Geometry: final body of the model. Coordinates: model frame, mm. Coordinates: 2 decimals unless noted, no trailing zeros. Write each loop counter-clockwise with the first axis right and the second up, starting at its lowest first coordinate (ties: lowest second). Pieces come first, ordered by that corner, then holes. Notation, with made-up numbers: (-9, 52.5) -> (34, 52.5) arc R17 ccw to (34, 83.5) -> close; hole circle Ø6 at (66, 74). An arc over 180 degrees is marked (long way). Answer as a JSON object with one key per item and string values. Group by question number.
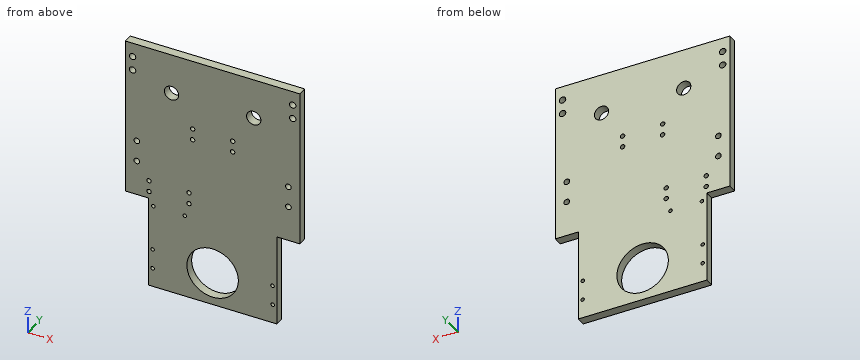
```python
from build123d import *

# Parameters (mm, degrees)
SKETCH1_W           = 122
SKETCH1_H           = 112
BOSS_EXTRUDE1_DEPTH = 6.2
SKETCH2_W           = 90
SKETCH2_H           = 65
BOSS_EXTRUDE2_DEPTH = 6.2
SKETCH3_R           = 1.25
SKETCH3_R_2         = 18
CUT_EXTRUDE1_DEPTH  = 136.648221514
SKETCH4_R           = 1.55
CUT_EXTRUDE2_DEPTH  = 136.648221514
SKETCH5_R           = 2
CUT_EXTRUDE3_DEPTH  = 10
SKETCH6_R           = 5
CUT_EXTRUDE4_DEPTH  = 10
SKETCH7_R           = 2.25
CUT_EXTRUDE5_DEPTH  = 136.648221514


with BuildPart() as part:
    # Sketch1 → Boss-Extrude1 (new body)
    with BuildSketch(Plane(origin=(0, 0, 0), x_dir=(1, 0, 0), z_dir=(0, 1, 0))):
        Rectangle(SKETCH1_W, SKETCH1_H)
    extrude(amount=BOSS_EXTRUDE1_DEPTH)

    # Sketch2 → Boss-Extrude2 (add)
    with BuildSketch(Plane(origin=(0, 0, 0), x_dir=(1, 0, 0), z_dir=(0, 1, 0))):
        with Locations((0, 88.5)):
            Rectangle(SKETCH2_W, SKETCH2_H)
    extrude(amount=BOSS_EXTRUDE2_DEPTH)

    # Sketch3 → Cut-Extrude1 (cut, through all)
    with BuildSketch(Plane(origin=(0, 6.2, 0), x_dir=(1, 0, 0), z_dir=(0, 1, 0))):
        with Locations(Location((-41.5, 61, 0), (0, 0, 270))):
            Circle(SKETCH3_R)
        with Locations(Location((-19.5, 61, 0), (0, 0, 270))):
            Circle(SKETCH3_R)
        with Locations(Location((-42, 93.5, 0), (0, 0, 270))):
            Circle(SKETCH3_R)
        with Locations(Location((-42, 107.5, 0), (0, 0, 270))):
            Circle(SKETCH3_R)
        with Locations(Location((42, 107.5, 0), (0, 0, 270))):
            Circle(SKETCH3_R)
        with Locations(Location((41.859469925, 93.5, 0), (0, 0, 270))):
            Circle(SKETCH3_R)
        with Locations(Location((0, 97.5, 0), (0, 0, 270))):
            Circle(SKETCH3_R_2)
    extrude(amount=-CUT_EXTRUDE1_DEPTH, mode=Mode.SUBTRACT)

    # Sketch4 → Cut-Extrude2 (cut, through all)
    with BuildSketch(Plane(origin=(0, 6.2, 0), x_dir=(1, 0, 0), z_dir=(0, 1, 0))):
        with Locations(Location((-44.5, 51, 0), (0, 0, 270))):
            Circle(SKETCH4_R)
        with Locations(Location((-16.5, 51, 0), (0, 0, 270))):
            Circle(SKETCH4_R)
        with Locations(Location((-16.5, 43, 0), (0, 0, 270))):
            Circle(SKETCH4_R)
        with Locations(Location((-44.5, 43, 0), (0, 0, 270))):
            Circle(SKETCH4_R)
        with Locations(Location((-14, 2.5, 0), (0, 0, 270))):
            Circle(SKETCH4_R)
        with Locations(Location((14, 2.5, 0), (0, 0, 270))):
            Circle(SKETCH4_R)
        with Locations(Location((14, -5.5, 0), (0, 0, 270))):
            Circle(SKETCH4_R)
        with Locations(Location((-14, -5.5, 0), (0, 0, 270))):
            Circle(SKETCH4_R)
    extrude(amount=-CUT_EXTRUDE2_DEPTH, mode=Mode.SUBTRACT)

    # Sketch5 → Cut-Extrude3 (cut)
    with BuildSketch(Plane(origin=(0, 6.2, 0), x_dir=(1, 0, 0), z_dir=(0, 1, 0))):
        with Locations(Location((-53, 31, 0), (0, 0, 270))):
            Circle(SKETCH5_R)
        with Locations(Location((-53, 16, 0), (0, 0, 270))):
            Circle(SKETCH5_R)
        with Locations(Location((53, 16, 0), (0, 0, 270))):
            Circle(SKETCH5_R)
        with Locations(Location((53, 31, 0), (0, 0, 270))):
            Circle(SKETCH5_R)
    extrude(amount=-CUT_EXTRUDE3_DEPTH, mode=Mode.SUBTRACT)

    # Sketch6 → Cut-Extrude4 (cut)
    with BuildSketch(Plane(origin=(0, 6.2, 0), x_dir=(1, 0, 0), z_dir=(0, 1, 0))):
        with Locations(Location((-28.75, -27.5, 0), (0, 0, 270))):
            Circle(SKETCH6_R)
        with Locations(Location((28.75, -27.5, 0), (0, 0, 270))):
            Circle(SKETCH6_R)
    extrude(amount=-CUT_EXTRUDE4_DEPTH, mode=Mode.SUBTRACT)

    # Sketch7 → Cut-Extrude5 (cut, through all)
    with BuildSketch(Plane(origin=(0, 6.2, 0), x_dir=(1, 0, 0), z_dir=(0, 1, 0))):
        with Locations(Location((-56, -36, 0), (0, 0, 270))):
            Circle(SKETCH7_R)
        with Locations(Location((-56, -46, 0), (0, 0, 270))):
            Circle(SKETCH7_R)
        with Locations(Location((56, -46, 0), (0, 0, 270))):
            Circle(SKETCH7_R)
        with Locations(Location((56, -36, 0), (0, 0, 270))):
            Circle(SKETCH7_R)
    extrude(amount=-CUT_EXTRUDE5_DEPTH, mode=Mode.SUBTRACT)


solid = part.part
```
Item 1: Section A-A on x = 0. Output: boundary loops of the cut face in (y, z), then the cut area to 3 significant figures.
Item 2: Contact query for flat-ended pins moving along their axis: pin 1 (3 mm diameter, centred on x = 42, z = -107.5, fed in from +Y); pin 2 (2.5 mm diameter, centred on x = 14, z = -2.5, fed in from -Y); pin 3 (1.9 mm diameter, centred on x = -55, y = 3.5, fed in from -Z). Output: stop coordinate, or through.
Item 3: Ray query, L1, parallel to X at y = 4.5, z = 27; L2, parallel to X at y = 1.75, z = -61; L3, parallel to X at y = 3, z = -92. Return the intervals inside material, ascending. Write a range as [from, to].
Item 4: Section B-B on y = 3.25. Give the number of separate pieces and of enclosed holes in the cut face, then the cut area to 3 significant figures.
Answer sheet:
{
 "1": {"outline": "(0, -121) -> (6.2, -121) -> (6.2, -115.5) -> (0, -115.5) -> close; (0, -79.5) -> (6.2, -79.5) -> (6.2, 56) -> (0, 56) -> close", "area": "874 mm^2"},
 "2": {"pin 1": "stops at y = 6.2", "pin 2": "passes through", "pin 3": "stops at z = -56"},
 "3": {"L1": "x = [-61, -33.72], [-23.78, 23.78], [33.72, 61]", "L2": "x = [-45, -42.75], [-40.25, -20.75], [-18.25, 45]", "L3": "x = [-45, -17.14], [17.14, 45]"},
 "4": {"separate pieces": "1", "enclosed holes": "25", "area": "18,100 mm^2"}
}
